Design review of the part built by this model. Coordinates are the model's own, in mm. A direction names the side the tool comes from. Give positions to 0.01 mm unless a question says otherwise; leave off trailing zeros. Order: outer loops, then holes, each group sorted by start corner. A loop starts at its lowest first (then second) coordinate and runs counter-clockwise, first axis right, second up. Notation, with made-up numbers: (7, 52) -> (59, 52) arc R35 cw to (59, 91) -> close; hole circle Ø6 at (48.5, -36.75). An arc over 180 degrees is marked (long way). Use a Markdown table: item, result. Add a question column.
```python
from build123d import *

# Parameters (mm, degrees)
F0_R     = 6.35
F1_DEPTH = 4.7625
F0_W     = 203.2
F0_H     = 101.6
F0_R_2   = 6.7945
F2_DEPTH = 6.35
F0_R_3   = 2.97688
F3_DEPTH = 4.7625
F4_DEPTH = 4.7625
F5_ANGLE = 270


with BuildPart() as f1:
    # F0 (on Top) → F1 (new body)
    with BuildSketch(Plane.XY):
        with BuildLine():
            Line((127, 88.16975), (76.2, 88.16975))
            ThreePointArc((76.2, 88.16975), (64.23025, 76.2), (76.2, 64.23025))
            Line((76.2, 64.23025), (127, 64.23025))
            ThreePointArc((127, 64.23025), (138.96975, 76.2), (127, 88.16975))
        make_face()
        with Locations((76.2, 76.2)):
            Circle(F0_R, mode=Mode.SUBTRACT)
        with Locations((101.6, 76.2)):
            Circle(F0_R, mode=Mode.SUBTRACT)
        with Locations((127, 76.2)):
            Circle(F0_R, mode=Mode.SUBTRACT)
    extrude(amount=F1_DEPTH)

    # F0 (on Top) → F2 (join)
    with BuildSketch(Plane.XY):
        with Locations((101.6, 50.8)):
            Rectangle(F0_W, F0_H)
        with Locations((19.05, 19.05)):
            Circle(F0_R_2, mode=Mode.SUBTRACT)
        with Locations((184.15, 19.05)):
            Circle(F0_R_2, mode=Mode.SUBTRACT)
        with BuildLine():
            ThreePointArc((76.2, 64.23025), (64.23025, 76.2), (76.2, 88.16975))
            Line((76.2, 88.16975), (127, 88.16975))
            ThreePointArc((127, 88.16975), (138.96975, 76.2), (127, 64.23025))
            Line((127, 64.23025), (76.2, 64.23025))
        make_face(mode=Mode.SUBTRACT)
    extrude(amount=F2_DEPTH)

    # F0 (on Top) → F3 (join)
    with BuildSketch(Plane.XY):
        with Locations((19.05, 19.05)):
            Circle(F0_R_2)
        with Locations((19.05, 19.05)):
            Circle(F0_R_3, mode=Mode.SUBTRACT)
    extrude(amount=F3_DEPTH)

    # F0 (on Top) → F4 (join)
    with BuildSketch(Plane.XY):
        with Locations((184.15, 19.05)):
            Circle(F0_R_2)
        with Locations((184.15, 19.05)):
            Circle(F0_R_3, mode=Mode.SUBTRACT)
    extrude(amount=F4_DEPTH)


with BuildPart() as f1_1:
    # F5: moved
    add(f1.part.rotate(Axis((0, 0, 3.175), (0, 0, -1)), F5_ANGLE))


with BuildPart() as f1_2:
    # F6: moved
    add(f1_1.part.moved(Location((101.6, 0, 0))))


solid = f1_2.part
```
1) Machinability: for faces 4 (the flat face through (50, 100, 0)), 5 (the cylindrical face through (25.663, 64.233, 5.545)), which of the approach directions +Z, -Z, +X, -X, +Y, -Y give a long, thin tool a straight path to every point of the face, cutting with its end or side? Answer none if there is none.
2) For L1, parallel to Y at x = 82.55, z = 1.3; L2, parallel to Y at x = 82.55, z = 5.3; L3, parallel to X at y = 101.6, z = 1.75, list the stretches that pass through material, from the lowest coordinate up. Write a range as [from, to].
3) Add section C-C (z = 3.25). Give the boundary of the cut face in (x, y).
4) Add section A-A (y = 19.05). Give the boundary of the cut face in (x, z), then the cut area to 3 significant figures.
5) Add section B-B (x = 25.4). Give the boundary of the cut face in (y, z).
6) Add section D-D (x = 82.55). Give the boundary of the cut face in (y, z).
7) The part is to be moulded in two halves that separate along X. For faces 1 (the flat face through (0, 100, 3)), 2 (the flat face through (52, 0, 3)), 3 (the cylindrical face through (25.137, 138.967, 5.545)), say which applies: +X half, -X half, draft (parallel to the pull), parting line (faces both ways), or undercut.
8) Insertion check: pin 1 (7 mm diameter, centred on x = 82, y = 22, fed in from +Z); pin 2 (7 mm diameter, centred on x = 82.55, y = 184.15, fed in from -Z). Each pin has a flat end and moves straight along its axis. Give the tip position at first contact, or say it passes through.
Worked answers:
| question | item | result |
|---|---|---|
| 1 | face 4 | -Z, +X, -X, +Y, -Y |
| 1 | face 5 | +Z |
| 2 | L1 | [0, 16.07], [22.03, 181.17], [187.13, 203.2] |
| 2 | L2 | [0, 12.26], [25.84, 177.36], [190.94, 203.2] |
| 2 | L3 | [0, 19.05], [31.75, 101.6] |
| 3 | outline | (0, 0) -> (101.6, 0) -> (101.6, 203.2) -> (0, 203.2) -> close; hole circle Ø12.7 at (25.4, 76.2); hole circle Ø12.7 at (25.4, 101.6); hole circle Ø12.7 at (25.4, 127); hole circle Ø5.95 at (82.55, 19.05); hole circle Ø5.95 at (82.55, 184.15) |
| 4 | outline | (0, 0) -> (79.57, 0) -> (79.57, 4.76) -> (75.76, 4.76) -> (75.76, 6.35) -> (0, 6.35) -> close; (85.53, 0) -> (101.6, 0) -> (101.6, 6.35) -> (89.34, 6.35) -> (89.34, 4.76) -> (85.53, 4.76) -> close |
| 4 | area | 595 mm^2 |
| 5 | outline | (0, 0) -> (69.85, 0) -> (69.85, 4.76) -> (64.23, 4.76) -> (64.23, 6.35) -> (0, 6.35) -> close; (82.55, 0) -> (95.25, 0) -> (95.25, 4.76) -> (82.55, 4.76) -> close; (107.95, 0) -> (120.65, 0) -> (120.65, 4.76) -> (107.95, 4.76) -> close; (133.35, 0) -> (203.2, 0) -> (203.2, 6.35) -> (138.97, 6.35) -> (138.97, 4.76) -> (133.35, 4.76) -> close |
| 6 | outline | (0, 0) -> (16.07, 0) -> (16.07, 4.76) -> (12.26, 4.76) -> (12.26, 6.35) -> (0, 6.35) -> close; (22.03, 0) -> (181.17, 0) -> (181.17, 4.76) -> (177.36, 4.76) -> (177.36, 6.35) -> (25.84, 6.35) -> (25.84, 4.76) -> (22.03, 4.76) -> close; (187.13, 0) -> (203.2, 0) -> (203.2, 6.35) -> (190.94, 6.35) -> (190.94, 4.76) -> (187.13, 4.76) -> close |
| 7 | face 1 | -X half |
| 7 | face 2 | draft |
| 7 | face 3 | undercut |
| 8 | pin 1 | z = 4.76 |
| 8 | pin 2 | z = 0 |
